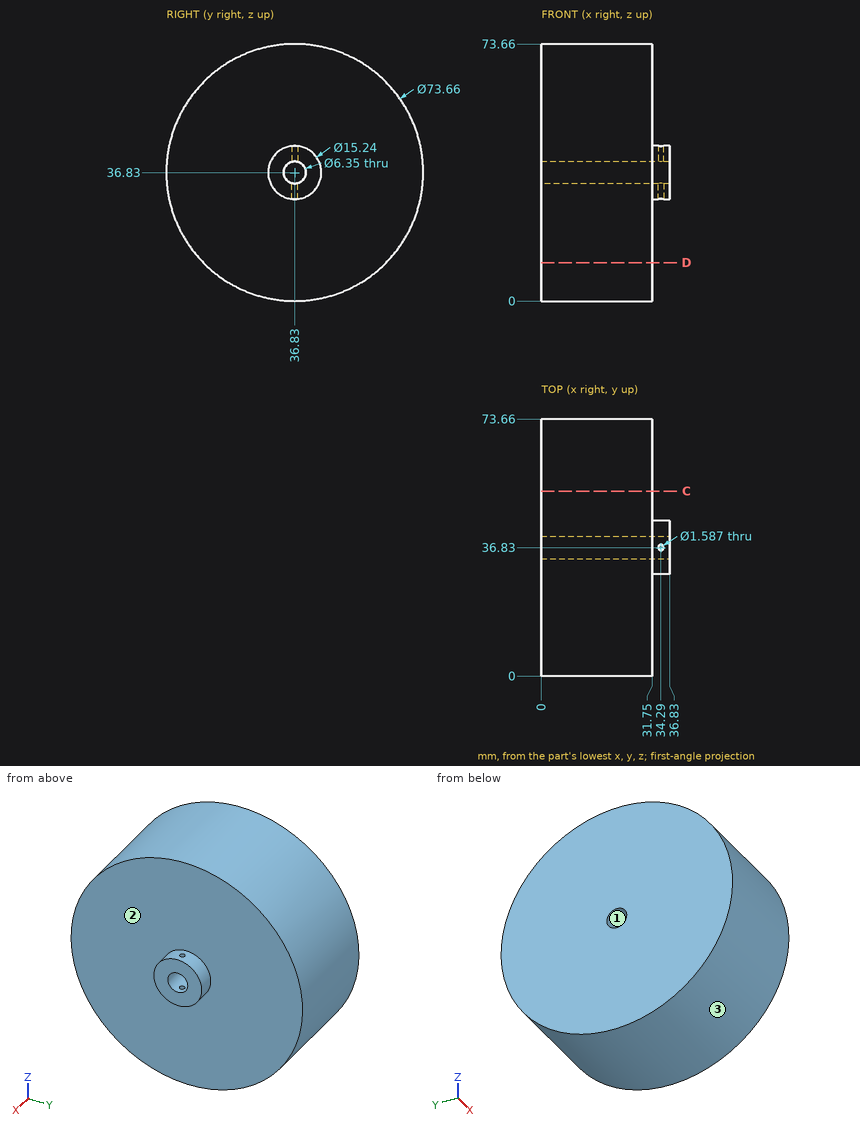
Could you check a few things on this drawing? It's one solid part, dimensions in mm from its lowest x, y, z. Give positions to 0.01 mm unless a question says otherwise; leave off trailing zeros. Loops run counter-clockwise (first coordinate to the right, second up) from the corner with the lowest first, then second, coordinate; pieces in that order, holes last. Notation, with made-up numbers: M 63.5,-1 L 83.5,-1 A25 ccw 83.5,38 Z; hole C 41.25,23.5 d9. An arc over 180 degrees is marked long. Answer as a JSON object with one key per item and string values.
Q1. If I drill on probe 1 along Y at (x, z) = (9, 36.83) (1 decimal); probe 2 along X at (y, z) = (69, 47); probe 3 along Y at (x, z) = (34, 42) (1 decimal), over which ranges is the centre line in solid material (lowest first)? Write a range as [from, to].
Values found:
{"probe 1": "y = [0, 33.7], [40, 73.7]", "probe 2": "x = [0, 31.75]", "probe 3": "y = [31.2, 36.1], [37.6, 42.4]"}
Q2. For P1, Ø1.5, axis at x = 26.5, y = 29.5, coming from the -Z side; P2, Ø12, axis at x = 18, y = 38, coming from the +Z side; P3, Ø1.8, axis at x = 34.29, y = 36.83, coming from the +Z side; P4, Ø5, axis at x = 23.5, y = 52.5, coming from the -Z side (1 decimal), each with a flat end and sliding along its axis, tell me the tip position at first contact or that it passes through.
Values found:
{"P1": "stops at z = 0.59", "P2": "stops at z = 73.66", "P3": "stops at z = 44.45", "P4": "stops at z = 2.4"}
Q3. Suppose I cut it at C-C, the plane y = 53. List the corners of the cut face in (x, z) for me, plus the area to 3 significant figures.
Values found:
{"outline": "M 0,3.74 L 31.75,3.74 L 31.75,69.92 L 0,69.92 Z", "area": "2,100 mm²"}
Q4. If we mould it in two halves opening along Y, with no side actions, what happens to the marked faces 1, 2 and 3? For each: pulls with the +Y half, pulls with the -Y half, needs draft (parallel to the pull), parting line crosses it, or undercut.
Values found:
{"face 1": "undercut", "face 2": "needs draft", "face 3": "parting line crosses it"}
Q5. Suppose I cut it at D-D, the plane z = 11. List the corners of the cut face in (x, y) for me.
Values found:
{"outline": "M 0,10.58 L 31.75,10.58 L 31.75,63.08 L 0,63.08 Z"}
